Source: CAD feature listing. Evaluate the final solid. Frame: model axes, mm. Give positions to 0.01 mm unless a question says otherwise; leave off trailing zeros. Write each loop counter-clockwise with the first axis right and the second up, starting at its lowest first coordinate (ties: lowest second). Pieces come first, ordered by that corner, then holes.
```python
from build123d import *

# Parameters (mm, degrees)
SKETCH1_R           = 24
BOSS_EXTRUDE1_DEPTH = 2
SKETCH2_R           = 3.25
SKETCH2_R_2         = 1.9
CUT_EXTRUDE1_DEPTH  = 3


with BuildPart() as part:
    # Sketch1 → Boss-Extrude1 (new body)
    with BuildSketch(Plane(origin=(0, 0, 0), x_dir=(1, 0, 0), z_dir=(0, 1, 0))):
        Circle(SKETCH1_R)
    extrude(amount=BOSS_EXTRUDE1_DEPTH)

    # Sketch2 → Cut-Extrude1 (cut, through all)
    with BuildSketch(Plane(origin=(0, 2, 0), x_dir=(1, 0, 0), z_dir=(0, 1, 0))):
        Circle(SKETCH2_R)
        with Locations((0, 8.85)):
            Circle(SKETCH2_R_2)
        with Locations((7.664324823, -4.425)):
            Circle(SKETCH2_R_2)
        with Locations((-7.664324823, -4.425)):
            Circle(SKETCH2_R_2)
        with Locations((0, 16.85)):
            Circle(SKETCH2_R_2)
    extrude(amount=-CUT_EXTRUDE1_DEPTH, mode=Mode.SUBTRACT)


solid = part.part
```
1. Section query B-B (x = 0). Return loops of the section in (y, z), plus the area to 3 significant figures.
2. Section query C-C (y = 1.1). Return loops of the section in (x, z) (3 decimals), plus the area to 3 significant figures.
3. Section query D-D (z = -8.85). Return loops of the section in (x, y), plus the area to 3 significant figures.
4. Pull-direction query (X, two-part tool) for faces 1 (the cylindrical face through (-23.977, 0.986, -1.055)), 2 (the flat face through (0, 2, 5)), 3 (the cylindrical face through (-9.065, 1.014, 3.141)); classes: pulls with the +X half, pulls with the -X half, needs draft (parallel to the pull), parting line crosses it, or undercut.
5. Line query: probe 1 along Z at (x, y) = (0, 0.9); probe 2 along X at (y, z) = (0.6, 5.5); probe 3 along X at (y, z) = (0.95, 4). Output: solid intervals per line, ascending.
6. Section query A-A (z = 0). Return loops of the section in (x, y), plus the area to 3 significant figures.
7. Pin query (flat end, axial travel): P1, Ø3.5, axis at x = -7.66, z = 4.42, coming from the -Y side; P2, Ø1, axis at x = 2.5, y = 0.5, coming from the +Z side. Return the tip coordinate at first contact, or that it passes through.
The answers:
1. outline: (0, -24) - (2, -24) - (2, -18.75) - (0, -18.75) - close; (0, -14.95) - (2, -14.95) - (2, -10.75) - (0, -10.75) - close; (0, -6.95) - (2, -6.95) - (2, -3.25) - (0, -3.25) - close; (0, 3.25) - (2, 3.25) - (2, 24) - (0, 24) - close
1. area: 67.8 mm2
2. outline: circle Ø48 at (0, 0); hole circle Ø3.8 at (-7.664, 4.425); hole circle Ø6.5 at (0, 0); hole circle Ø3.8 at (0, -16.85); hole circle Ø3.8 at (0, -8.85); hole circle Ø3.8 at (7.664, 4.425)
2. area: 1,730 mm2
3. outline: (-22.31, 0) - (-1.9, 0) - (-1.9, 2) - (-22.31, 2) - close; (1.9, 0) - (22.31, 0) - (22.31, 2) - (1.9, 2) - close
3. area: 81.6 mm2
4. face 1: parting line crosses it
4. face 2: needs draft
4. face 3: undercut
5. probe 1: z = -24 to -18.75, -14.95 to -10.75, -6.95 to -3.25, 3.25 to 24
5. probe 2: x = -23.36 to -9.23, -6.1 to 6.1, 9.23 to 23.36
5. probe 3: x = -23.66 to -9.52, -5.81 to 5.81, 9.52 to 23.66
6. outline: (-24, 0) - (-3.25, 0) - (-3.25, 2) - (-24, 2) - close; (3.25, 0) - (24, 0) - (24, 2) - (3.25, 2) - close
6. area: 83.0 mm2
7. P1: passes through
7. P2: stops at z = 23.92
